Autodesk Inventor part; units mm, degrees
ref_plane "YZ Plane" through (0, 0, 0) normal (1, 0, 0) x (0, 1, 0)
ref_plane "XZ Plane" through (0, 0, 0) normal (0, 1, 0) x (-1, 0, 0)
ref_plane "XY Plane" through (0, 0, 0) normal (0, 0, 1) x (1, 0, 0)
sketch "Sketch1" plane through (0, 0, 0) normal (0, 1, 0) x (-1, 0, 0)
  circle A0 centre (0, 0) radius 2.3876
  arc A1 (2.9591, 0) -> (1.8161, -2.3362) centre (0, 0) ccw
  line L0 (2.9591, 0) -> (2.3876, 0)
  line L1 (1.8161, -2.3362) -> (1.8161, -17.78)
  line L2 (1.8161, -17.78) -> (2.9591, -17.78)
  line L3 (2.9591, -17.78) -> (2.9591, 0)
  dimension "d0" = 4.7752
  dimension "d1" = 5.9182
  dimension "d2" = 17.78
  dimension "d3" = 1.143
extrude "Extrusion1" add sketch "Sketch1" along normal blind 38.1
sketch "Sketch2" plane through (0, 38.1, 0) normal (0, 1, 0) x (1, 0, 0)
  line L0 (-4.1424, -3.452) -> (4.5842, -3.452)
  line L1 (4.5842, -3.452) -> (4.5842, 3.3967)
  line L2 (4.5842, 3.3967) -> (-4.1424, 3.3967)
  line L3 (-4.1424, 3.3967) -> (-4.1424, -3.452)
  point P0 (0, 0)
  dimension "d6" = 8.7266
  dimension "d7" = 6.8487
  dimension "d8" = 4.5842
  dimension "d9" = 3.3967
sketch "Sketch3" plane through (0, 0, 0) normal (0, -1, 0) x (1, 0, 0)
  line L0 (-4.1424, -3.3967) -> (-4.1424, 3.452)
  line L1 (-4.1424, 3.452) -> (4.5842, 3.452)
  line L2 (4.5842, 3.452) -> (4.5842, -3.3967)
  line L3 (4.5842, -3.3967) -> (-4.1424, -3.3967)
  point P0 (0, 0)
extrude "Extrusion2" cut sketch "Sketch3" against normal blind 10.16
extrude "Extrusion3" cut sketch "Sketch2" against normal blind 10.16
sketch "Sketch4" plane through (-1.8161, 0, -3.7778) normal (1, 0, 0) x (0, 0, -1)
  circle A0 centre (7.6522, 5.08) radius 2.54
  circle A1 centre (7.6522, 33.02) radius 2.54
  line L0 (14.0022, 0) -> (14.0022, 38.1)
  line L1 (0, 0) -> (14.0022, 0)
  line L2 (0, 38.1) -> (14.0022, 38.1)
  line L3 (14.0022, 0) -> (14.0022, 38.1)
  line L4 (-0.381, 38.1) -> (14.0022, 38.1)
  line L5 (-0.381, 0) -> (14.0022, 0)
  point P0 (-2.3362, 0)
  dimension "d17" = 6.35
  dimension "d16" = 5.08
  dimension "d15" = 5.08
  dimension "d14" = 5.08
  dimension "d21" = 14.0022
  dimension "d22" = 14.0022
  dimension "d23" = 16.3385
  dimension "d24" = 38.1
extrude "Extrusion4" cut sketch "Sketch4" against normal up to next
equation "\"d14\" = d16"
properties part number "Hinge Wall 1"
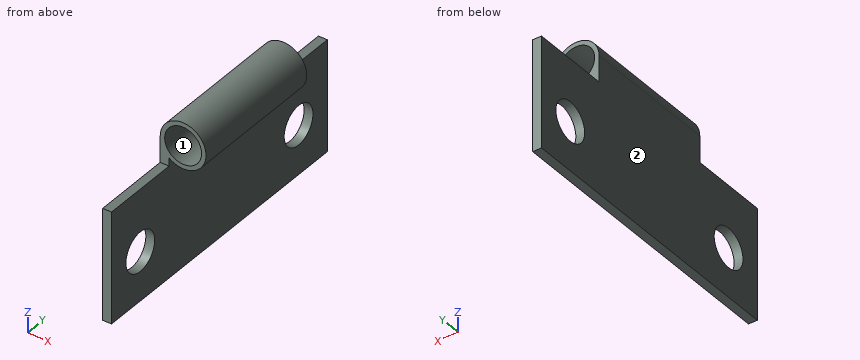
The model under review builds one solid part; all positions refer to its coordinate system, in mm. Face numbers are marked on the shaded views. Round coordinates to 2 decimals unless told otherwise and drop trailing zeros. Write each loop counter-clockwise with the first axis right and the second up, starting at its lowest first coordinate (ties: lowest second). Pieces come first, ordered by that corner, then holes. Notation, with made-up numbers: M 48,16 L 98,16 A6 cw 98,21 Z; hole C 56,57.25 d1. An arc over 180 degrees is marked long. Answer as CSV lines item,"result". Start each with the question number.
Q1. Wall thickness on line 1 along Y through (x, z) = (-2.2, -11.43); line 2 along X through (y, z) = (14.75, 0); line 3 along X through (y, z) = (24, -8): over which ranges is each line inside the solid? List them lowest first.
Q2. Consider section D-D, the plane y = 19. Give the boundary of the cut face in (x, z), then the cut area to 3 significant figures.
Q3. The part is to be moulded in two halves that separate along X. For the marked faces 1 and 2, say which applies: +X half, -X half, draft (parallel to the pull), parting line (faces both ways), or undercut.
Q4. Consider section B-B, the plane y = 5.08. Give the boundary of the cut face in (x, z).
Q5. Clearance check with flat-ended pins moving along their axes: P1, Ø10, axis at y = 24, z = -14, coming from the +X side; P2, Ø1.3, axis at x = -2.5, y = 34.5, coming from the +Z side; P3, Ø4, axis at y = 33.02, z = -11.43, coming from the -X side. State where each tip first meets the part, or that it passes through.
Q6. Consider section A-A, the plane z = -11.43. Give the boundary of the cut face in (x, y), then the cut area to 3 significant figures.
Q7. Consider section C-C, the plane x = 0.35. Give the boundary of the cut face in (y, z).
Result set:
1,line 1,"y = 0 to 2.54, 7.62 to 30.48, 35.56 to 38.1"
1,line 2,"x = -2.96 to -2.39, 2.39 to 2.96"
1,line 3,"x = -2.96 to -1.82"
2,outline,"M -2.96,-17.78 L -1.82,-17.78 L -1.82,-2.34 A2.96 ccw long -2.96,0 Z; hole C 0,0 d4.78"
2,area,"28.1 mm²"
3,face 1,"undercut"
3,face 2,"-X half"
4,outline,"M -2.96,-17.78 L -1.82,-17.78 L -1.82,-13.97 L -2.96,-13.97 Z; M -2.96,-8.89 L -1.82,-8.89 L -1.82,-3.4 L -2.96,-3.4 Z"
5,P1,"stops at x = -1.82"
5,P2,"stops at z = -3.4"
5,P3,"passes through"
6,outline,"M -2.96,0 L -1.82,0 L -1.82,2.54 L -2.96,2.54 Z; M -2.96,7.62 L -1.82,7.62 L -1.82,30.48 L -2.96,30.48 Z; M -2.96,35.56 L -1.82,35.56 L -1.82,38.1 L -2.96,38.1 Z"
6,area,"31.9 mm²"
7,outline,"M 10.16,-2.94 L 27.94,-2.94 L 27.94,-2.36 L 10.16,-2.36 Z; M 10.16,2.36 L 27.94,2.36 L 27.94,2.94 L 10.16,2.94 Z"
